from build123d import *

# Parameters (mm, degrees)
F1_DEPTH = 25.4
F2_DEPTH = 54.61407
F3_W     = 19.551679
F3_H     = 57.516087
F4_DEPTH = 26.09864
F5_R     = 7.652629
F5_R_2   = 7.80409
F6_DEPTH = 25.4


with BuildPart() as f1:
    # F0 (on Top) → F1 (new body)
    with BuildSketch(Plane.XY):
        with BuildLine():
            ThreePointArc((-29.517332, 0), (-37.88477, 20.200783), (-58.085553, 28.568221))
            Line((-58.085553, 28.568221), (-58.085553, 16.098264))
            ThreePointArc((-58.085553, 16.098264), (-46.702362, 11.383191), (-41.98729, 0))
            ThreePointArc((-41.98729, 0), (-46.702362, -11.383191), (-58.085553, -16.098264))
            Line((-58.085553, -16.098264), (-58.085553, -28.568221))
            ThreePointArc((-58.085553, -28.568221), (-37.88477, -20.200783), (-29.517332, 0))
        make_face()
        with BuildLine():
            Line((-58.085553, 16.098264), (-58.085553, 28.568221))
            ThreePointArc((-58.085553, 28.568221), (-86.653775, 0), (-58.085553, -28.568221))
            Line((-58.085553, -28.568221), (-58.085553, -16.098264))
            ThreePointArc((-58.085553, -16.098264), (-74.183817, 0), (-58.085553, 16.098264))
        make_face()
        with BuildLine():
            Line((58.085553, 28.568221), (-58.085553, 28.568221))
            ThreePointArc((-58.085553, 28.568221), (-37.88477, 20.200783), (-29.517332, 0))
            ThreePointArc((-29.517332, 0), (-37.88477, -20.200783), (-58.085553, -28.568221))
            Line((-58.085553, -28.568221), (58.085553, -28.568221))
            Line((58.085553, -28.568221), (58.085553, 28.568221))
        make_face()
    extrude(amount=F1_DEPTH)

    # F0 (on Top) → F2 (join)
    with BuildSketch(Plane.XY):
        with BuildLine():
            Line((-58.085553, 16.098264), (-58.085553, 28.568221))
            ThreePointArc((-58.085553, 28.568221), (-86.653775, 0), (-58.085553, -28.568221))
            Line((-58.085553, -28.568221), (-58.085553, -16.098264))
            ThreePointArc((-58.085553, -16.098264), (-74.183817, 0), (-58.085553, 16.098264))
        make_face()
        with BuildLine():
            ThreePointArc((-29.517332, 0), (-37.88477, 20.200783), (-58.085553, 28.568221))
            Line((-58.085553, 28.568221), (-58.085553, 16.098264))
            ThreePointArc((-58.085553, 16.098264), (-46.702362, 11.383191), (-41.98729, 0))
            ThreePointArc((-41.98729, 0), (-46.702362, -11.383191), (-58.085553, -16.098264))
            Line((-58.085553, -16.098264), (-58.085553, -28.568221))
            ThreePointArc((-58.085553, -28.568221), (-37.88477, -20.200783), (-29.517332, 0))
        make_face()
    extrude(amount=F2_DEPTH)

    # F3 (on face) → F4 (join)
    with BuildSketch(Plane.XY):
        with Locations((48.208024, 0.189823)):
            Rectangle(F3_W, F3_H)
    extrude(amount=-F4_DEPTH)

    # F5 (on face) → F6 (cut)
    with BuildSketch(Plane.YZ.offset(57.983864)):
        with Locations((-14.27424, -13.706455)):
            Circle(F5_R)
        with Locations((15.358331, -14.498299)):
            Circle(F5_R_2)
    extrude(amount=-F6_DEPTH, mode=Mode.SUBTRACT)


solid = f1.part
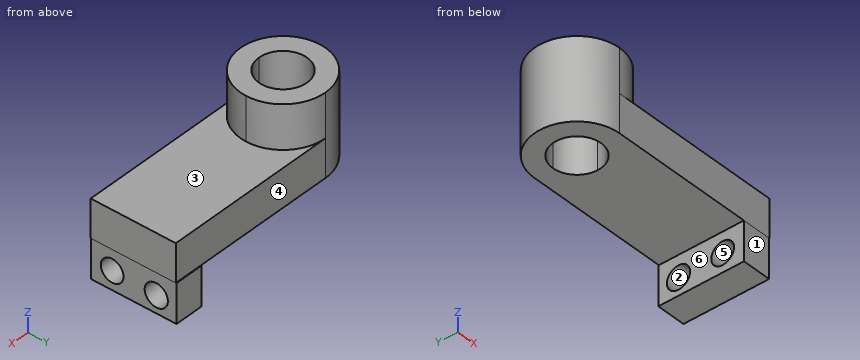
Input: part model. Units: mm. Frame: model coordinates. Face numbers are marked on the shaded views. A direction names the side the tool comes from. Give positions to 0.01 mm unless a question says otherwise; leave off trailing zeros. Loops run counter-clockwise (first coordinate to the right, second up) from the corner with the lowest first, then second, coordinate; pieces in that order, holes last. Notation, with made-up numbers: M 61,-14 L 117,-14 A20 cw 117,-8 Z; hole C 65.25,67 d10. An arc over 180 degrees is marked long. Use CSV: the item, a comma, the result in double quotes.
(1) Section A-A, the plane y = -11. Return loops of the section in (x, z), plus the area to 3 significant figures.
Outcome:
outline,"M -84.45,0 L -69.84,0 L -69.84,54.61 L -84.45,54.61 Z; M -46.33,0 L 38.43,0 L 38.43,-6.79 L 57.98,-6.79 L 57.98,0 L 58.09,0 L 58.09,25.4 L -31.72,25.4 L -31.72,54.61 L -46.33,54.61 Z; M 38.43,-26.1 L 57.98,-26.1 L 57.98,-20.62 L 38.43,-20.62 Z"
area,"4,120 mm²"
(2) Pin query (flat end, axial travel): P1, Ø12, axis at x = 15, y = -3, coming from the -Z side; P2, Ø17.5, axis at y = -14.27, z = -13.71, coming from the -X side; P3, Ø5, axis at y = 10, z = 3.5, coming from the -X side. Return the tip coordinate at first contact, or that it passes through.
Outcome:
P1,"stops at z = 0"
P2,"stops at x = 38.43"
P3,"stops at x = -85.65"
(3) Section D-D, the plane x = 45. Return loops of the section in (y, z), plus the area to 3 significant figures.
Outcome:
outline,"M -28.57,-26.1 L 28.95,-26.1 L 28.95,0 L 28.57,0 L 28.57,25.4 L -28.57,25.4 Z; hole C -14.27,-13.71 d15.31; hole C 15.36,-14.5 d15.61"
area,"2,580 mm²"
(4) Set-up query: the marked faces 4, 5 and 6. Return all of +Z, -Z, +X, -X, +Y, -Y with unobstructed straight access to the full face (end or side cutting, diameter ignored); none if empty.
Outcome:
face 4,"+Z, +X, -X, +Y"
face 5,"+X, -X"
face 6,"-Z, -X, +Y, -Y"
(5) Pull-direction query (Y, two-part tool) for the marked faces 1, 2 and 3; classes: pulls with the +Y half, pulls with the -Y half, needs draft (parallel to the pull), parting line crosses it, or undercut.
Outcome:
face 1,"pulls with the -Y half"
face 2,"undercut"
face 3,"needs draft"
(6) Material intervals for L1, parallel to Y at x = -57.5, z = 19; L2, parallel to Y at x = -21.5, z = 4; L3, parallel to Z at x = -31.5, y = 8, sorted ascending. Write a range as [from, to].
Outcome:
L1,"y = [-28.57, -16.09], [16.09, 28.57]"
L2,"y = [-28.57, 28.57]"
L3,"z = [0, 54.61]"
(7) Section C-C, the plane z = 33. Return loops of the section in (x, y), plus the area to 3 significant figures.
Outcome:
outline,"M -58.09,-28.57 A28.57 ccw -29.52,0 A28.57 ccw -58.09,28.57 A28.57 ccw Z; hole M -58.09,-16.1 A16.1 ccw -58.09,16.1 A16.1 ccw Z"
area,"1,750 mm²"
(8) Section B-B, the plane x = -47.5. Return loops of the section in (y, z).
Outcome:
outline,"M -28.57,0 L -12.13,0 L -12.13,54.61 L -26.53,54.61 L -26.53,25.4 L -28.57,25.4 Z; M 12.13,0 L 28.57,0 L 28.57,25.4 L 26.53,25.4 L 26.53,54.61 L 12.13,54.61 Z"
